Source: CAD feature listing. Evaluate the final solid. Frame: model axes, mm. Round coordinates to 2 decimals unless told otherwise and drop trailing zeros. Write each loop counter-clockwise with the first axis right and the second up, starting at its lowest first coordinate (ties: lowest second). Pieces come first, ordered by that corner, then holes. Notation, with made-up numbers: M -26,28.25 L 20,28.25 A24 cw 20,64.25 Z; hole C 3,74.25 d11. An arc over 180 degrees is marked long. Answer in a Markdown table with one row per item. Add a question column.
Item 1: Cut plane B-B on z = 2.55. Return loops of the section in (x, y) (3 decimals), and give its area (3 significant figures).
Item 2: Cut plane A-A on y = 76. Return loops of the section in (x, z) (3 decimals).
Item 3: Cut plane D-D on x = 0. Return loops of the section in (y, z) (3 decimals).
Item 4: Contact query for flat-ended pins moving along their axis: pin 1 (2 mm diameter, centred on y = -29.5, z = 1.5, fed in from -X); pin 2 (2 mm diameter, centred on x = 80.5, z = 3, fed in from -Y); pin 3 (3 mm diameter, centred on x = 0, y = 76, fed in from +Z); pin 4 (2 mm diameter, centred on x = -59, z = 1, fed in from -Y). Output: stop coordinate, or through.
Item 5: Material intervals for probe 1 along Y at (x, z) = (0, 1.25) (3 decimals); probe 2 along Y at (x, z) = (83.5, 2.65) (3 decimals); probe 3 along X at (y, z) = (-47.5, 3.15), sorted ascending.
Item 6: Cut plane C-C on x = 83.5. Return loops of the section in (y, z) (3 decimals), and give its area (3 significant figures).
from build123d import *

# Parameters (mm, degrees)
SKETCH1_R           = 2.525
BOSS_EXTRUDE1_DEPTH = 4


with BuildPart() as part:
    # Sketch1 → Boss-Extrude1 (new body)
    with BuildSketch(Plane.XY):
        with BuildLine():
            Line((-43.5, 86), (-43.5, 46))
            Line((-43.5, 46), (-63.5, 46))
            ThreePointArc((-63.5, 46), (-70.571067812, 43.071067812), (-73.5, 36))
            Line((-73.5, 36), (-73.5, 16))
            Line((-73.5, 16), (-93.5, 16))
            Line((-93.5, 16), (-93.5, -16))
            Line((-93.5, -16), (-73.5, -16))
            Line((-73.5, -16), (-73.5, -36))
            ThreePointArc((-73.5, -36), (-70.571067812, -43.071067812), (-63.5, -46))
            Line((-63.5, -46), (-43.5, -46))
            Line((-43.5, -46), (-43.5, -66))
            Line((-43.5, -66), (43.5, -66))
            Line((43.5, -66), (43.5, -46))
            Line((43.5, -46), (63.5, -46))
            ThreePointArc((63.5, -46), (70.571067812, -43.071067812), (73.5, -36))
            Line((73.5, -36), (73.5, -16))
            Line((73.5, -16), (93.5, -16))
            Line((93.5, -16), (93.5, 16))
            Line((93.5, 16), (73.5, 16))
            Line((73.5, 16), (73.5, 36))
            ThreePointArc((73.5, 36), (70.571067812, 43.071067812), (63.5, 46))
            Line((63.5, 46), (43.5, 46))
            Line((43.5, 46), (43.5, 86))
            Line((43.5, 86), (-43.5, 86))
        make_face()
        with Locations((0, 76)):
            Circle(SKETCH1_R, mode=Mode.SUBTRACT)
        with Locations((-83.5, 0)):
            Circle(SKETCH1_R, mode=Mode.SUBTRACT)
        with Locations((83.5, 0)):
            Circle(SKETCH1_R, mode=Mode.SUBTRACT)
        with Locations((0, -56)):
            Circle(SKETCH1_R, mode=Mode.SUBTRACT)
    extrude(amount=BOSS_EXTRUDE1_DEPTH)


solid = part.part
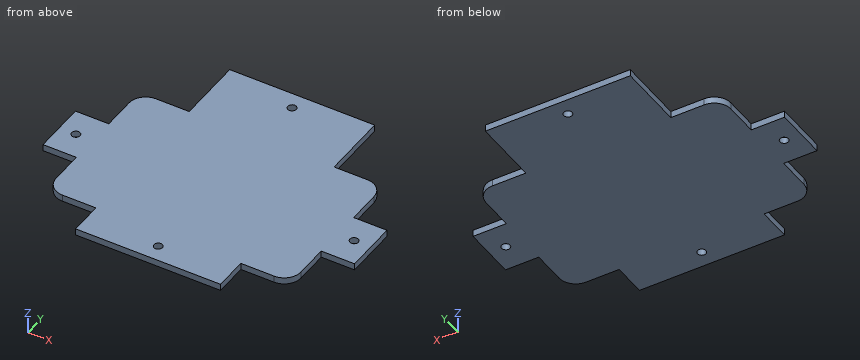
Results below:
| question | item | result |
|---|---|---|
| 1 | outline | M -93.5,-16 L -73.5,-16 L -73.5,-36 A10 ccw -63.5,-46 L -43.5,-46 L -43.5,-66 L 43.5,-66 L 43.5,-46 L 63.5,-46 A10 ccw 73.5,-36 L 73.5,-16 L 93.5,-16 L 93.5,16 L 73.5,16 L 73.5,36 A10 ccw 63.5,46 L 43.5,46 L 43.5,86 L -43.5,86 L -43.5,46 L -63.5,46 A10 ccw -73.5,36 L -73.5,16 L -93.5,16 Z; hole C -83.5,0 d5.05; hole C 0,-56 d5.05; hole C 0,76 d5.05; hole C 83.5,0 d5.05 |
| 1 | area | 19,900 mm2 |
| 2 | outline | M -43.5,0 L -2.525,0 L -2.525,4 L -43.5,4 Z; M 2.525,0 L 43.5,0 L 43.5,4 L 2.525,4 Z |
| 3 | outline | M -66,0 L -58.525,0 L -58.525,4 L -66,4 Z; M -53.475,0 L 73.475,0 L 73.475,4 L -53.475,4 Z; M 78.525,0 L 86,0 L 86,4 L 78.525,4 Z |
| 4 | pin 1 | x = -73.5 |
| 4 | pin 2 | y = -16 |
| 4 | pin 3 | through |
| 4 | pin 4 | y = -46 |
| 5 | probe 1 | -66 to -58.525, -53.475 to 73.475, 78.525 to 86 |
| 5 | probe 2 | -16 to -2.525, 2.525 to 16 |
| 5 | probe 3 | -43.5 to 43.5 |
| 6 | outline | M -16,0 L -2.525,0 L -2.525,4 L -16,4 Z; M 2.525,0 L 16,0 L 16,4 L 2.525,4 Z |
| 6 | area | 108 mm2 |
